from build123d import *

# Parameters (mm, degrees)
ESQUISSE1_R             = 2.5
BASE_EXTRUSION_DEPTH    = 2
BASE_EXTRUSION_TAPER    = 4
CONG_1_R                = 1
ESQUISSE2_R             = 2
BOSS_EXTRU_1_DEPTH      = 6
ESQUISSE3_R             = 1.5
BOSS_EXTRU_2_DEPTH      = 8
CHANFREIN1_SIZE         = 0.5
ENL_V_MAT_EXTRU_1_DEPTH = 1
ESQUISSE5_W             = 0.75
ESQUISSE5_H             = 5.593358395
ENL_V_MAT_EXTRU_2_DEPTH = 0.5


with BuildPart() as part:
    # Esquisse1 → Base-Extrusion (new body)
    with BuildSketch(Plane.XY):
        Circle(ESQUISSE1_R)
    extrude(amount=BASE_EXTRUSION_DEPTH, taper=BASE_EXTRUSION_TAPER)

    # Congé1
    cong_1_edges = [part.edges().sort_by_distance(p)[0] for p in [
        (-2.360146376, 0, 2),
    ]]
    fillet(cong_1_edges, radius=CONG_1_R)

    # Esquisse2 → Boss.-Extru.1 (add)
    with BuildSketch(Plane(origin=(0, 0, 0), x_dir=(-1, 0, 0), z_dir=(0, 0, -1))):
        Circle(ESQUISSE2_R)
    extrude(amount=BOSS_EXTRU_1_DEPTH)

    # Esquisse3 → Boss.-Extru.2 (add)
    with BuildSketch(Plane(origin=(0, 0, -6), x_dir=(-1, 0, 0), z_dir=(0, 0, -1))):
        Circle(ESQUISSE3_R)
    extrude(amount=BOSS_EXTRU_2_DEPTH)

    # Chanfrein1
    chanfrein1_edges = [part.edges().sort_by_distance(p)[0] for p in [
        (1.5, 0, -14),
    ]]
    chamfer(chanfrein1_edges, length=CHANFREIN1_SIZE)

    # Esquisse4 → Enlèv. mat.-Extru.1 (cut)
    with BuildSketch(Plane.XY.offset(2)):
        with BuildLine():
            Line((-1.75, -0.375), (-0.75, -0.375))
            ThreePointArc((-0.75, -0.375), (-0.592927061, -0.592927061), (-0.375, -0.75))
            Line((-0.375, -0.75), (-0.375, -1.75))
            Line((-0.375, -1.75), (0.375, -1.75))
            Line((0.375, -1.75), (0.375, -0.75))
            ThreePointArc((0.375, -0.75), (0.592927061, -0.592927061), (0.75, -0.375))
            Line((0.75, -0.375), (1.75, -0.375))
            Line((1.75, -0.375), (1.75, 0.375))
            Line((1.75, 0.375), (0.75, 0.375))
            ThreePointArc((0.75, 0.375), (0.592927061, 0.592927061), (0.375, 0.75))
            Line((0.375, 0.75), (0.375, 1.75))
            Line((0.375, 1.75), (-0.375, 1.75))
            Line((-0.375, 1.75), (-0.375, 0.75))
            ThreePointArc((-0.375, 0.75), (-0.592927061, 0.592927061), (-0.75, 0.375))
            Line((-0.75, 0.375), (-1.75, 0.375))
            Line((-1.75, 0.375), (-1.75, -0.375))
        make_face()
    extrude(amount=-ENL_V_MAT_EXTRU_1_DEPTH, mode=Mode.SUBTRACT)

    # Esquisse5 → Enlèv. mat.-Extru.2 (cut)
    with BuildSketch(Plane.XY.offset(2)):
        with Locations((0, -0.203384651)):
            Rectangle(ESQUISSE5_W, ESQUISSE5_H)
    extrude(amount=-ENL_V_MAT_EXTRU_2_DEPTH, mode=Mode.SUBTRACT)


solid = part.part
Model file for the job. Use its own axes, mm. A direction names the side the tool comes from. Give positions to 0.01 mm unless a question says otherwise; leave off trailing zeros. Write each loop counter-clockwise with the first axis right and the second up, starting at its lowest first coordinate (ties: lowest second). Pieces come first, ordered by that corner, then holes. Notation, with made-up numbers: (42.5, -5) -> (70.5, -5) arc R18 cw to (70.5, 5) -> close; hole circle Ø9 at (15, 46.5). An arc over 180 degrees is marked (long way). Write item = value, one per line.
(1) Slice it at A-A, the plane x = 0. Give the cut face in (y, z), then the cut area to 3 significant figures.
Determined:
outline = (-2.5, 0) -> (-2, 0) -> (-2, -6) -> (-1.5, -6) -> (-1.5, -13.5) -> (-1, -14) -> (1, -14) -> (1.5, -13.5) -> (1.5, -6) -> (2, -6) -> (2, 0) -> (2.5, 0) -> (2.43, 1.07) arc R1 ccw to (2.29, 1.5) -> (1.75, 1.5) -> (1.75, 1) -> (-1.75, 1) -> (-1.75, 1.5) -> (-2.29, 1.5) arc R1 ccw to (-2.43, 1.07) -> close
area = 53.3 mm2
(2) Slice it at D-D, the plane z = -4.5. Give the cut face in (x, y).
Determined:
outline = circle Ø4 at (0, 0)
(3) Probe line 1 along Y through (x, z) = (-0.9, 1.25) (3 decimals); line 2 along Z through (x, y) = (0, 0.65); line 3 along X through (y, z) = (-0.75, -5.5). List the from-to ranges inside material, lowest first.
Determined:
line_1 = -2.22 to -0.375, 0.375 to 2.22
line_2 = -14 to 1
line_3 = -1.85 to 1.85
(4) Tool access for faces 4 (the face through (-1, 2, 0)), 5 (the face through (0.375, -1.3, 1.5)), 6 (the face through (0.8, -0.8, 2)): list every direction of +Z, -Z, +X, -X, +Y, -Y with a clear straight run to the whole face (end or side of a thin tool).
Determined:
face_4 = -Z
face_5 = +Z
face_6 = +Z, +X, -X, +Y, -Y
(5) Slice it at C-C, the plane z = -10.75. Give the cut face in (x, y).
Determined:
outline = circle Ø3 at (0, 0)
(6) Slice it at B-B, the plane y = 0. Give the cut face in (x, z).
Determined:
outline = (-2.5, 0) -> (-2, 0) -> (-2, -6) -> (-1.5, -6) -> (-1.5, -13.5) -> (-1, -14) -> (1, -14) -> (1.5, -13.5) -> (1.5, -6) -> (2, -6) -> (2, 0) -> (2.5, 0) -> (2.43, 1.07) arc R1 ccw to (1.75, 1.95) -> (1.75, 1) -> (-1.75, 1) -> (-1.75, 1.95) arc R1 ccw to (-2.43, 1.07) -> close
(7) Mould opens along Y. For faces 1 (the face through (0, -2, -3)), 2 (the face through (0, 0, -14)), 3 (the face through (0, 0, 1)) say: released by +Y, released by -Y, zero draft, split by the parting line, or undercut.
Determined:
face_1 = split by the parting line
face_2 = zero draft
face_3 = undercut
(8) Flat gauge pins, fed straight in: P1, Ø0.6, axis at x = 0, y = 2, coming from the +Z side; P2, Ø0.8, axis at y = 0, z = 1.5, coming from the -X side; P3, Ø1.1, axis at x = 1, z = 1.5, coming from the -Y side. Where does each tip first touch, or does it go through?
Determined:
P1 = 1.5
P2 = -2.42
P3 = -2.35
